Source: CAD feature listing. Evaluate the final solid. Frame: model axes, mm. A direction names the side the tool comes from. Coordinates: 2 decimals unless noted, no trailing zeros. Order: outer loops, then holes, each group sorted by start corner. A loop starts at its lowest first (then second) coordinate and runs counter-clockwise, first axis right, second up. Notation, with made-up numbers: (-29.75, 27.5) - (22.25, 27.5) arc R17 ccw to (22.25, 47.5) - close; hole circle Ø10 at (-25.5, -33). An arc over 180 degrees is marked (long way). One line per question, with ' | ' between items. Start each with the question number.
(1) Draft query along Z for faces 4 (the flat face through (-1, 89, 82.5)), 5 (the flat face through (-98.5, 89, 1)), 6 (the flat face through (-1, 89, -82.5)), 7 (the cylindrical face through (67.71, 172.4, 65.7)). Return one class per face: +Z half, -Z half, draft (parallel to the pull), parting line (faces both ways), or undercut.
(2) Access query for faces 1 (the flat face through (-74, 173, 50.551)), 2 (the flat face through (-47.815, 173, 67)), 3 (the cylindrical face through (-73.641, 172.395, 60.936)). Directions: +Z, -Z, +X, -X, +Y, -Y. A direction counts if a zero-diameter tool reaches every point of the face in a straight line with its end or side. Return the directions, or none.
(3) Section A-A (x = 82.5). Return the cut outline in (y, z).
(4) Contact query for flat-ended pins moving along their axis: P1, Ø4.5, axis at x = 70.5, y = 170.5, coming from the +Z side; P2, Ø7.5, axis at y = 172.5, z = 69.5, coming from the -X side; P3, Ø4.5, axis at y = 175, z = 64, coming from the +X side. Output: stop coordinate, or through.
from build123d import *

# Parameters (mm, degrees)
SKETCH_2_W          = 197
SKETCH_2_H          = 165
EXTRUDE_1_DEPTH     = 180
SKETCH_3_W          = 50.684983536
SKETCH_3_H          = 31.949298514
CUT_EXTRUDE_2_DEPTH = 15
SKETCH_4_W          = 51.160754844
SKETCH_4_H          = 30.284098936
CUT_EXTRUDE_3_DEPTH = 15
SKETCH_5_R          = 5.238888092
EXTRUDE_2_DEPTH     = 15
SKETCH_6_R          = 5.653498574
EXTRUDE_3_DEPTH     = 15


with BuildPart() as part:
    # 草图2 → 凸台-拉伸1 (new body)
    with BuildSketch(Plane(origin=(0, 0, 0), x_dir=(1, 0, 0), z_dir=(0, 1, 0))):
        Rectangle(SKETCH_2_W, SKETCH_2_H)
    extrude(amount=EXTRUDE_1_DEPTH)

    # 草图3 → 切除-拉伸2 (cut)
    with BuildSketch(Plane(origin=(0, 180, 0), x_dir=(1, 0, 0), z_dir=(0, 1, 0))):
        with Locations((-73.157508232, -66.525350743)):
            Rectangle(SKETCH_3_W, SKETCH_3_H)
    extrude(amount=-CUT_EXTRUDE_2_DEPTH, mode=Mode.SUBTRACT)

    # 草图4 → 切除-拉伸3 (cut)
    with BuildSketch(Plane(origin=(0, 180, 0), x_dir=(1, 0, 0), z_dir=(0, 1, 0))):
        with Locations((72.919622578, -67.357950532)):
            Rectangle(SKETCH_4_W, SKETCH_4_H)
    extrude(amount=-CUT_EXTRUDE_3_DEPTH, mode=Mode.SUBTRACT)

    # 草图5 → 凸台-拉伸2 (add)
    with BuildSketch(Plane(origin=(0, 165, 0), x_dir=(1, 0, 0), z_dir=(0, 1, 0))):
        with Locations(Location((-75.647637988, -65.775383345, 0), (0, 0, 90))):
            Circle(SKETCH_5_R)
    extrude(amount=EXTRUDE_2_DEPTH)

    # 草图6 → 凸台-拉伸3 (add)
    with BuildSketch(Plane(origin=(0, 165, 0), x_dir=(1, 0, 0), z_dir=(0, 1, 0))):
        with Locations(Location((73.228131145, -66.927099699, 0), (0, 0, 270))):
            Circle(SKETCH_6_R)
    extrude(amount=EXTRUDE_3_DEPTH)


solid = part.part
Response values:
1) face 4: +Z half | face 5: draft | face 6: -Z half | face 7: undercut
2) face 1: -X, +Y | face 2: +Z, +Y | face 3: +Y
3) outline: (0, -82.5) - (180, -82.5) - (180, 52.22) - (165, 52.22) - (165, 82.5) - (0, 82.5) - close
4) P1: stops at z = 72.56 | P2: stops at x = -80.89 | P3: stops at x = 78.84
